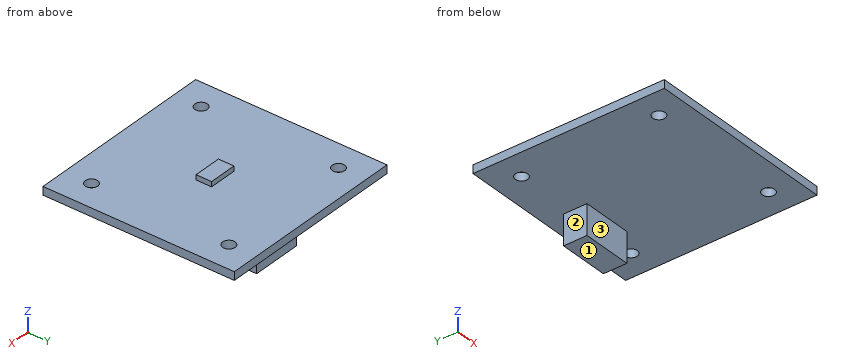
from build123d import *

# Parameters (mm, degrees)
SKIZZE1_W                       = 38.3
SKIZZE1_H                       = 38.3
SKIZZE1_R                       = 1.25
AUFSATZ_LINEAR_AUSTRAGEN1_DEPTH = 1.65
SKIZZE2_W                       = 5.6
SKIZZE2_H                       = 3.1
AUFSATZ_LINEAR_AUSTRAGEN2_DEPTH = 1
SKETCH2_W                       = 10
SKETCH2_H                       = 4.7
BOSS_EXTRUDE1_DEPTH             = 6


with BuildPart() as part:
    # Skizze1 → Aufsatz-Linear austragen1 (new body)
    with BuildSketch(Plane.XY):
        Rectangle(SKIZZE1_W, SKIZZE1_H)
        with Locations((-13.75, 13.75)):
            Circle(SKIZZE1_R, mode=Mode.SUBTRACT)
        with Locations((13.75, 13.75)):
            Circle(SKIZZE1_R, mode=Mode.SUBTRACT)
        with Locations((13.75, -13.75)):
            Circle(SKIZZE1_R, mode=Mode.SUBTRACT)
        with Locations((-13.75, -13.75)):
            Circle(SKIZZE1_R, mode=Mode.SUBTRACT)
    extrude(amount=AUFSATZ_LINEAR_AUSTRAGEN1_DEPTH)

    # Skizze2 → Aufsatz-Linear austragen2 (add)
    with BuildSketch(Plane.XY.offset(1.65)):
        Rectangle(SKIZZE2_W, SKIZZE2_H)
    extrude(amount=AUFSATZ_LINEAR_AUSTRAGEN2_DEPTH)

    # Sketch2 → Boss-Extrude1 (add)
    with BuildSketch(Plane(origin=(0, 0, 0), x_dir=(-1, 0, 0), z_dir=(0, 0, -1))):
        with Locations((-3.55, 12.8)):
            Rectangle(SKETCH2_W, SKETCH2_H)
    extrude(amount=BOSS_EXTRUDE1_DEPTH)


solid = part.part
Model file for the job. Use its own axes, mm. Face numbers are marked on the shaded views. A direction names the side the tool comes from. Round coordinates to 2 decimals unless told otherwise and drop trailing zeros. Loops run counter-clockwise (first coordinate to the right, second up) from the corner with the lowest first, then second, coordinate; pieces in that order, holes last. Notation, with made-up numbers: (88.5, 44.25) - (118.5, 44.25) arc R22 ccw to (118.5, 56.25) - close; hole circle Ø2 at (74, 24). An arc over 180 degrees is marked (long way). Write each question's results on one line, items separated by ' | '.
(1) Saw through at D-D, the plane x = 8. List the corners of the cut face in (y, z).
Answer below:
outline: (-19.15, 0) - (10.45, 0) - (10.45, -6) - (15.15, -6) - (15.15, 0) - (19.15, 0) - (19.15, 1.65) - (-19.15, 1.65) - close
(2) Wall check: L1, parallel to Y at x = -13.75, z = 0.85; L2, parallel to X at y = 14, z = -1; L3, parallel to Z at x = 3, y = -1.5. Give the ranges that are in metal, low to high.
Answer below:
L1: y = -19.15 to -15, -12.5 to 12.5, 15 to 19.15 | L2: x = -1.45 to 8.55 | L3: z = 0 to 1.65
(3) Saw through at C-C, the plane y = 13.75. List the corners of the cut face in (x, z), then the cut area to 3 significant figures.
Answer below:
outline: (-19.15, 0) - (-15, 0) - (-15, 1.65) - (-19.15, 1.65) - close; (-12.5, 0) - (-1.45, 0) - (-1.45, -6) - (8.55, -6) - (8.55, 0) - (12.5, 0) - (12.5, 1.65) - (-12.5, 1.65) - close; (15, 0) - (19.15, 0) - (19.15, 1.65) - (15, 1.65) - close | area: 115 mm^2
(4) Pin check, flat tips, straight feed: pin 1 (0.8 mm diameter, centred on y = 0.5, z = 2.5, fed in from +X); pin 2 (1.1 mm diameter, centred on x = -1, z = 2, fed in from +Y); pin 3 (1.4 mm diameter, centred on y = 11.5, z = -2.5, fed in from -X); pin 4 (10 mm diameter, centred on x = 1.5, y = 2, fed in from -Z). Stop position of each tip, or through.
Answer below:
pin 1: stops at x = 2.8 | pin 2: stops at y = 19.15 | pin 3: stops at x = -1.45 | pin 4: stops at z = 0
(5) 3-axis set-ups, long thin cutter, end or side, ignore diameter. For the marked faces 1, 2 and 3: which of +Z, -Z, +X, -X, +Y, -Y reach the whole face in a straight line?
Answer below:
face 1: -Z, +X, -X, +Y, -Y | face 2: -Z, -X, +Y, -Y | face 3: -Z, +X, -X, -Y
(6) Saw through at A-A, the plane y = -13. List the corners of the cut face in (x, z).
Answer below:
outline: (-19.15, 0) - (-14.75, 0) - (-14.75, 1.65) - (-19.15, 1.65) - close; (-12.75, 0) - (12.75, 0) - (12.75, 1.65) - (-12.75, 1.65) - close; (14.75, 0) - (19.15, 0) - (19.15, 1.65) - (14.75, 1.65) - close
(7) Saw through at B-B, the plane x = -13.75. List the corners of the cut face in (y, z), then the cut area to 3 significant figures.
Answer below:
outline: (-19.15, 0) - (-15, 0) - (-15, 1.65) - (-19.15, 1.65) - close; (-12.5, 0) - (12.5, 0) - (12.5, 1.65) - (-12.5, 1.65) - close; (15, 0) - (19.15, 0) - (19.15, 1.65) - (15, 1.65) - close | area: 54.9 mm^2
